Can you work these out from the model? Positions are in its coordinate system, mm. A direction names the side the tool comes from. Coordinates: 2 decimals unless noted, no trailing zeros. Order: outer loops, then holes, each group sorted by start corner. A loop starts at its lowest first (then second) coordinate and runs counter-clockwise, first axis right, second up. Notation, with made-up numbers: (-34.75, -13.75) -> (3.25, -13.75) arc R9 ccw to (3.25, -6.75) -> close; hole circle Ø7 at (-31, 81). An arc over 180 degrees is marked (long way). Use a Markdown table: item, result. Add a question column.
1. Suppose I cut it at B-B, the plane z = 62.5. State how many separate pieces and enclosed holes the cut face has, then the cut area to 3 significant figures.
2. We'd pull the mould along Y, two halves only. Please class faces 1 (the flat face through (-27.5, 0, 258)), 2 (the flat face through (-30, 0, 259)), 3 (the flat face through (24, -30, 242)): pulls with the +Y half, pulls with the -Y half, needs draft (parallel to the pull), parting line crosses it, or undercut.
3. Suppose I cut it at A-A, the plane y = 1.5. List the corners of the cut face in (x, z) for me, then the cut area to 3 significant figures.
4. If I drill on line 1 along X through (y, z) = (15.5, 359.5); line 2 along Y through (x, z) = (24.5, 63); line 3 along Y through (x, z) = (25, 115), over which ranges is the centre line in solid material (lowest first)? Write a range as from..to.
5. For pin 1 Ø3 at (x, z) = (-13.5, 394) entering from +Y; pin 2 Ø6 at (x, y) = (15, 15) entering from +Z; pin 3 Ø12 at (x, y) = (-10.5, 17) entering from +Z, each with a flat end and sliding along its axis, tell me the tip position at first contact or that it passes through.
6. For faces 4 (the flat face through (27.5, 0, 241)), 5 (the flat face through (24, 30, 242)), which set-ups out of +Z, -Z, +X, -X, +Y, -Y let a thin tool reach every point of the face, with its end or its side?
```python
from build123d import *

# Parameters (mm, degrees)
F0_R          = 3
F0_R_2        = 2.5
F1_DEPTH      = 500
F2_R          = 2
F3_R          = 7
F6_DEPTH      = 30
F6_DEPTH_BACK = 30


# Not quite as in the source:
# - a feature names something its author has since deleted; it is built from what else it names


with BuildPart() as f1:
    # F0 (on Top) → F1 (new body)
    with BuildSketch(Plane.XY):
        with BuildLine():
            Line((18.15, -30), (30, -30))
            Line((30, -30), (30, -18.15))
            Line((30, -18.15), (27.5, -18.15))
            Line((27.5, -18.15), (27.5, -20.15))
            Line((27.5, -20.15), (21.5477069044, -20.15))
            ThreePointArc((21.5477069044, -20.15), (19.5, -15), (21.5477069044, -9.85))
            Line((21.5477069044, -9.85), (27.5, -9.85))
            Line((27.5, -9.85), (27.5, -11.85))
            Line((27.5, -11.85), (30, -11.85))
            Line((30, -11.85), (30, 11.85))
            Line((30, 11.85), (27.5, 11.85))
            Line((27.5, 11.85), (27.5, 9.85))
            Line((27.5, 9.85), (21.5477069044, 9.85))
            ThreePointArc((21.5477069044, 9.85), (19.5, 15), (21.5477069044, 20.15))
            Line((21.5477069044, 20.15), (27.5, 20.15))
            Line((27.5, 20.15), (27.5, 18.15))
            Line((27.5, 18.15), (30, 18.15))
            Line((30, 18.15), (30, 30))
            Line((30, 30), (18.15, 30))
            Line((18.15, 30), (18.15, 27.5))
            Line((18.15, 27.5), (20.15, 27.5))
            Line((20.15, 27.5), (20.15, 21.5477069044))
            ThreePointArc((20.15, 21.5477069044), (15, 19.5), (9.85, 21.5477069044))
            Line((9.85, 21.5477069044), (9.85, 27.5))
            Line((9.85, 27.5), (11.85, 27.5))
            Line((11.85, 27.5), (11.85, 30))
            Line((11.85, 30), (-11.85, 30))
            Line((-11.85, 30), (-11.85, 27.5))
            Line((-11.85, 27.5), (-9.85, 27.5))
            Line((-9.85, 27.5), (-9.85, 21.5477069044))
            ThreePointArc((-9.85, 21.5477069044), (-15, 19.5), (-20.15, 21.5477069044))
            Line((-20.15, 21.5477069044), (-20.15, 27.5))
            Line((-20.15, 27.5), (-18.15, 27.5))
            Line((-18.15, 27.5), (-18.15, 30))
            Line((-18.15, 30), (-30, 30))
            Line((-30, 30), (-30, 18.15))
            Line((-30, 18.15), (-27.5, 18.15))
            Line((-27.5, 18.15), (-27.5, 20.15))
            Line((-27.5, 20.15), (-21.5477069044, 20.15))
            ThreePointArc((-21.5477069044, 20.15), (-19.5, 15), (-21.5477069044, 9.85))
            Line((-21.5477069044, 9.85), (-27.5, 9.85))
            Line((-27.5, 9.85), (-27.5, 11.85))
            Line((-27.5, 11.85), (-30, 11.85))
            Line((-30, 11.85), (-30, -11.85))
            Line((-30, -11.85), (-27.5, -11.85))
            Line((-27.5, -11.85), (-27.5, -9.85))
            Line((-27.5, -9.85), (-21.5477069044, -9.85))
            ThreePointArc((-21.5477069044, -9.85), (-19.5, -15), (-21.5477069044, -20.15))
            Line((-21.5477069044, -20.15), (-27.5, -20.15))
            Line((-27.5, -20.15), (-27.5, -18.15))
            Line((-27.5, -18.15), (-30, -18.15))
            Line((-30, -18.15), (-30, -30))
            Line((-30, -30), (-18.15, -30))
            Line((-18.15, -30), (-18.15, -27.5))
            Line((-18.15, -27.5), (-20.15, -27.5))
            Line((-20.15, -27.5), (-20.15, -21.5477069044))
            ThreePointArc((-20.15, -21.5477069044), (-15, -19.5), (-9.85, -21.5477069044))
            Line((-9.85, -21.5477069044), (-9.85, -27.5))
            Line((-9.85, -27.5), (-11.85, -27.5))
            Line((-11.85, -27.5), (-11.85, -30))
            Line((-11.85, -30), (11.85, -30))
            Line((11.85, -30), (11.85, -27.5))
            Line((11.85, -27.5), (9.85, -27.5))
            Line((9.85, -27.5), (9.85, -21.5477069044))
            ThreePointArc((9.85, -21.5477069044), (15, -19.5), (20.15, -21.5477069044))
            Line((20.15, -21.5477069044), (20.15, -27.5))
            Line((20.15, -27.5), (18.15, -27.5))
            Line((18.15, -27.5), (18.15, -30))
        make_face()
        with Locations((-25, -25)):
            Circle(F0_R, mode=Mode.SUBTRACT)
        with Locations((-15, -15)):
            Circle(F0_R_2, mode=Mode.SUBTRACT)
        with Locations((25, -25)):
            Circle(F0_R, mode=Mode.SUBTRACT)
        with Locations((15, -15)):
            Circle(F0_R_2, mode=Mode.SUBTRACT)
        with Locations((-25, 25)):
            Circle(F0_R, mode=Mode.SUBTRACT)
        with Locations((-15, 15)):
            Circle(F0_R_2, mode=Mode.SUBTRACT)
        Polygon((-7, 22), (-7, 27.5), (0, 27.5), (7, 27.5), (7, 22), (10, 16), (10, 10), (16, 10), (22, 7), (27.5, 7), (27.5, 0), (27.5, -7), (22, -7), (16, -10), (10, -10), (10, -16), (7, -22), (7, -27.5), (0, -27.5), (-7, -27.5), (-7, -22), (-10, -16), (-10, -10), (-16, -10), (-22, -7), (-27.5, -7), (-27.5, 0), (-27.5, 7), (-22, 7), (-16, 10), (-10, 10), (-10, 16), align=None, mode=Mode.SUBTRACT)
        with Locations((15, 15)):
            Circle(F0_R_2, mode=Mode.SUBTRACT)
        with Locations((25, 25)):
            Circle(F0_R, mode=Mode.SUBTRACT)
    extrude(amount=F1_DEPTH)

    # F2
    f2_edges = [f1.edges().sort_by_distance(p)[0] for p in [
        (-7, 27.5, 250),
        (7, 27.5, 250),
    ]]
    fillet(f2_edges, radius=F2_R)

    # F3
    f3_edges = [f1.edges().sort_by_distance(p)[0] for p in [
        (-10, 16, 250),
        (10, 16, 250),
    ]]
    fillet(f3_edges, radius=F3_R)

    # F5 (on Front) → F6 (cut, two sides)
    with BuildSketch(Plane.XZ) as f6_sk:
        Polygon((190.5190290352, 666.216575566), (10.1971706169, 702.0848233142), (-30, 500), (150.3218584183, 464.1317522517), align=None)
        Polygon((-47.8999755124, -188.0671773906), (30, 0), (-147.6190188423, 73.5722065399), (-225.5189943547, -114.4949708507), align=None)
    extrude(amount=F6_DEPTH, mode=Mode.SUBTRACT)
    extrude(f6_sk.sketch, amount=-F6_DEPTH_BACK, mode=Mode.SUBTRACT)


solid = f1.part
```
Worked out:
| question | item | result |
|---|---|---|
| 1 | separate pieces | 1 |
| 1 | enclosed holes | 9 |
| 1 | area | 1,080 mm² |
| 2 | face 1 | undercut |
| 2 | face 2 | needs draft |
| 2 | face 3 | pulls with the -Y half |
| 3 | outline | (-30, 24.85) -> (-27.5, 23.82) -> (-27.5, 499.5) -> (-30, 500) -> close; (27.5, 1.04) -> (30, 0) -> (30, 488.07) -> (27.5, 488.56) -> close |
| 3 | area | 2,410 mm² |
| 4 | line 1 | x = -19.52..-17.45, -12.55..-9.9, 9.9..12.55, 17.45..19.52 |
| 4 | line 2 | y = -30..-27.96, -22.04..-20.15, -9.85..-7, 7..9.85, 20.15..22.04, 27.96..30 |
| 4 | line 3 | y = -30..-28, -22..-20.15, -9.85..-7, 7..9.85, 20.15..22, 28..30 |
| 5 | pin 1 | stops at y = 20.13 |
| 5 | pin 2 | stops at z = 491.65 |
| 5 | pin 3 | stops at z = 497.31 |
| 6 | face 4 | +Z, -Z |
| 6 | face 5 | +Z, -Z, +X, -X, +Y |
